```python
from build123d import *

# Parameters (mm, degrees)
BOSS_EXTRUDE1_DEPTH           = 8
M4_CLEARANCE_HOLE1_AT_2_COUNT = 2
M4_CLEARANCE_HOLE1_AT_2_PITCH = 112
SKETCH7_R                     = 3
CUT_EXTRUDE1_DEPTH            = 10
CUT_EXTRUDE1_DEPTH_BACK       = 6


with BuildPart() as part:
    # Sketch1 → Boss-Extrude1 (new body)
    with BuildSketch(Plane(origin=(0, 0, 0), x_dir=(0, 0, -1), z_dir=(1, 0, 0))):
        with BuildLine():
            Line((-60.995543931, 1.9), (-50.764456069, 1.9))
            ThreePointArc((-50.764456069, 1.9), (0, 50.8), (50.764456069, 1.9))
            Line((50.764456069, 1.9), (61.004456069, 1.9))
            Line((61.004456069, 1.9), (61.004456069, 16.9))
            Line((61.004456069, 16.9), (55.320249457, 16.9))
            ThreePointArc((55.320249457, 16.9), (54.442787227, 17.18342282), (53.896915423, 17.926586621))
            ThreePointArc((53.896915423, 17.926586621), (0, 56.8), (-53.896915423, 17.926586621))
            ThreePointArc((-53.896915423, 17.926586621), (-54.442787227, 17.18342282), (-55.320249457, 16.9))
            Line((-55.320249457, 16.9), (-60.995543931, 16.9))
            Line((-60.995543931, 16.9), (-60.995543931, 1.9))
        make_face()
    extrude(amount=BOSS_EXTRUDE1_DEPTH)

    # Sketch4 → M4 Clearance Hole1 (revolve, cut)
    with BuildSketch(Plane(origin=(4, 16.9, -56.004456069), x_dir=(0, 0, 1), z_dir=(1, 0, 0))):
        Polygon((0, 0), (0, 17.291850331), (2.15, 16), (2.15, 0), align=None)
    m4_clearance_hole1 = revolve(axis=Axis((4, 23.25, -56.004456069), (0, -1, 0)), mode=Mode.SUBTRACT)

    # M4 Clearance Hole1 at 2: M4 Clearance Hole1 ×2
    with Locations(*[(0, 0, i * M4_CLEARANCE_HOLE1_AT_2_PITCH) for i in range(1, M4_CLEARANCE_HOLE1_AT_2_COUNT)]):
        add(m4_clearance_hole1, mode=Mode.SUBTRACT)

    # Sketch7 → Cut-Extrude1 (cut, two sides)
    with BuildSketch(Plane(origin=(0, 16.9, 0), x_dir=(1, 0, 0), z_dir=(0, 1, 0))) as cut_extrude1_sk:
        with Locations((4, 56.004456069)):
            Circle(SKETCH7_R)
        with Locations((4, -55.995543931)):
            Circle(SKETCH7_R)
    extrude(amount=CUT_EXTRUDE1_DEPTH, mode=Mode.SUBTRACT)
    extrude(cut_extrude1_sk.sketch, amount=-CUT_EXTRUDE1_DEPTH_BACK, mode=Mode.SUBTRACT)


solid = part.part
```
Can you work these out from the model? Positions are in its coordinate system, mm. A direction names the side the tool comes from. Coordinates: 2 decimals unless noted, no trailing zeros. Loops run counter-clockwise (first coordinate to the right, second up) from the corner with the lowest first, then second, coordinate; pieces in that order, holes last. Notation, with made-up numbers: (32, 6) - (68, 6) arc R20 cw to (68, 37) - close; hole circle Ø9 at (56, 21.25). An arc over 180 degrees is marked (long way). Use a Markdown table: item, result.
Item 1: If I drill on probe 1 along Z at (x, y) = (4, 13); probe 2 along Z at (x, y) = (1.5, 14); probe 3 along Z at (x, y) = (6, 46), over which ranges is the centre line in solid material (lowest first)? Write a range as from..to.
Numbers:
| item | result |
|---|---|
| probe 1 | z = -61..-59, -53..-49.11, 49.11..53, 59..61 |
| probe 2 | z = -61..-57.66, -54.35..-48.83, 48.83..54.34, 57.65..61 |
| probe 3 | z = -33.32..-21.56, 21.56..33.32 |
Item 2: We'd pull the mould along X, two halves only. Please class faces 4 (the face through (8, 52, 0)), 5 (the face through (4, 10, 60.996)), 6 (the face through (5.3, 10.9, -54)), 7 (the face through (0, 52, 0)): released by +X, released by -X, zero draft, split by the parting line, or undercut.
Numbers:
| item | result |
|---|---|
| face 4 | released by +X |
| face 5 | zero draft |
| face 6 | undercut |
| face 7 | released by -X |
Item 3: I want a section at D-D on z = 0. Please give me the cut outline in (x, y), and give its area (3 significant figures).
Numbers:
| item | result |
|---|---|
| outline | (0, 50.8) - (8, 50.8) - (8, 56.8) - (0, 56.8) - close |
| area | 48.0 mm2 |
Item 4: I want a section at B-B on y = 6. Please give me the cut outline in (x, z), and give its area (3 significant figures).
Numbers:
| item | result |
|---|---|
| outline | (0, -61) - (8, -61) - (8, -50.44) - (0, -50.44) - close; (0, 50.44) - (8, 50.44) - (8, 61) - (0, 61) - close; hole circle Ø4.3 at (4, -56); hole circle Ø4.3 at (4, 56) |
| area | 140 mm2 |
Item 5: For faces 1 (the face through (3.9, 16.9, 59.4)), 2 (the face through (3.61, 14.68, 53.02)), 3 (the face through (3.9, 16.9, -59.5)), which set-ups out of +Z, -Z, +X, -X, +Y, -Y let a thin tool reach every point of the face, with its end or its side?
Numbers:
| item | result |
|---|---|
| face 1 | +Z, +X, -X, +Y |
| face 2 | +Y |
| face 3 | -Z, +X, -X, +Y |
Item 6: I want a section at C-C on y = 48.5. Please give me the cut outline in (x, z), and give its area (3 significant figures).
Numbers:
| item | result |
|---|---|
| outline | (0, -29.56) - (8, -29.56) - (8, -15.11) - (0, -15.11) - close; (0, 15.11) - (8, 15.11) - (8, 29.56) - (0, 29.56) - close |
| area | 231 mm2 |
Item 7: Will these pins go through, and if not, where does the flat tip stop? pin 1 (1.7 mm diameter, centred on x = 3.5, z = -58.5, fed in from +Y); pin 2 (3 mm diameter, centred on x = 1.5, y = 19, fed in from +Z); pin 3 (2 mm diameter, centred on x = 4, z = 10, fed in from -Y).
Numbers:
| item | result |
|---|---|
| pin 1 | stops at y = 16.9 |
| pin 2 | stops at z = 54.12 |
| pin 3 | stops at y = 49.59 |
